Source: three-view drawing plus pictorial views. Frame: mm from the lowest corner of the part. A direction names the side the tool comes from. Give positions to 0.01 mm unless a question says otherwise; leave off trailing zeros. Order: outer loops, then holes, each group sorted by start corner. A loop starts at its lowest first (then second) coordinate and runs counter-clockwise, first axis right, second up. Notation, with made-up numbers: M 38.5,87 L 64.5,87 A23 ccw 64.5,115 Z; hole C 85.5,74 d5. An arc over 180 degrees is marked long. One line per item, written item: value. Start each with the question number.
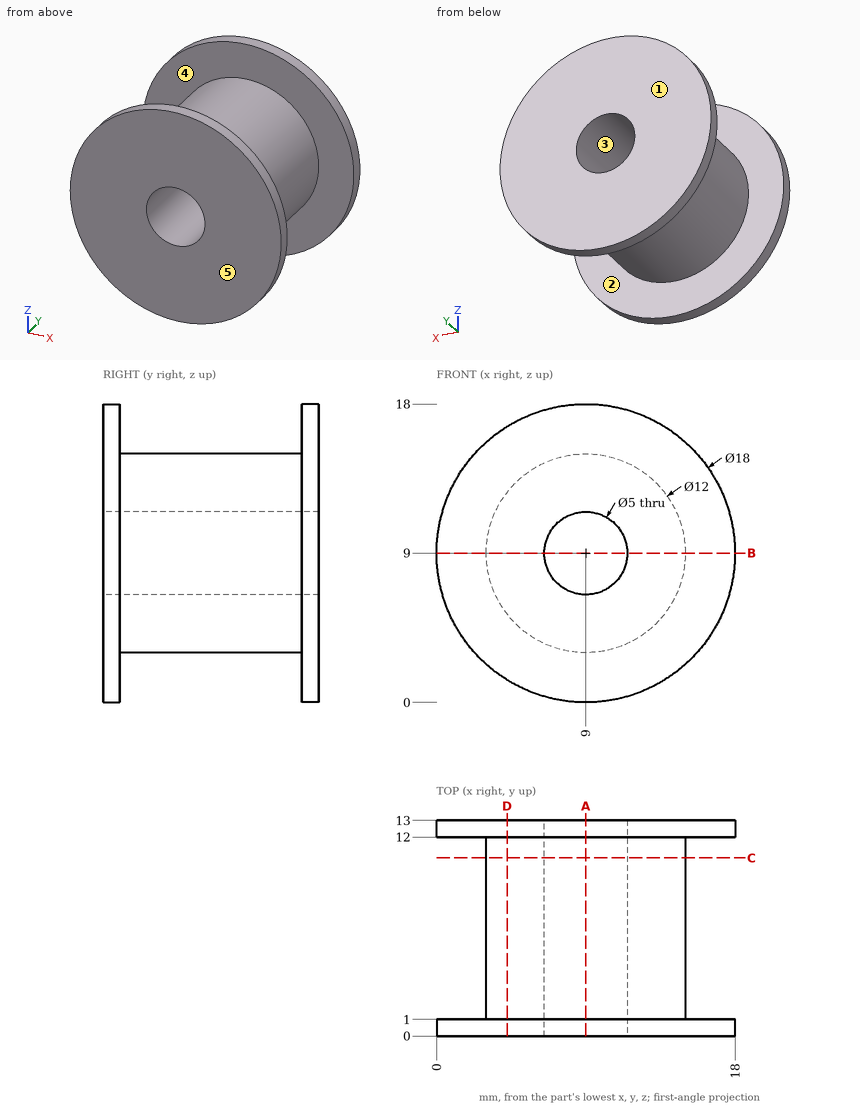
Q1. Set-up query: the marked faces 1 and 2. Return all of +Z, -Z, +X, -X, +Y, -Y with unobstructed straight access to the full face (end or side cutting, diameter ignored); none if empty.
Q2. Section query B-B on z = 9. Return loops of the section in (x, y).
Q3. Mould query, pull axis Y, two halves, no side actions, for the marked faces 3, 4 and 5. Classes: +Y half, -Y half, draft (parallel to the pull), parting line (faces both ways), or undercut.
Q4. Section query D-D on x = 4.25. Return loops of the section in (y, z), and give its area (3 significant figures).
Q5. Contact query for flat-ended pins moving along their axis: pin 1 (5 mm diameter, centred on x = 14.5, y = 10, fed in from -Z); pin 2 (4 mm diameter, centred on x = 4.5, y = 9.5, fed in from +Z); pin 3 (1.5 mm diameter, centred on y = 9.5, z = 4, fed in from +X). Output: stop coordinate, or through.
Q6. Ray query, line 1 along Y through (x, z) = (3.5, 12.75); line 2 along Z through (x, y) = (9, 3.75); line 3 along Z through (x, y) = (10, 2.25). Return the intervals inside material, ascending. Write a range as [from, to].
Q7. Section query C-C on y = 10.75. Return loops of the section in (x, z).
Q8. Section query A-A on x = 9. Return loops of the section in (y, z), and give its area (3 significant figures).
Results below:
1. face 1: +Z, -Z, +X, -X, +Y
1. face 2: none
2. outline: M 0,0 L 6.5,0 L 6.5,13 L 0,13 L 0,12 L 3,12 L 3,1 L 0,1 Z; M 11.5,0 L 18,0 L 18,1 L 15,1 L 15,12 L 18,12 L 18,13 L 11.5,13 Z
3. face 3: draft
3. face 4: undercut
3. face 5: -Y half
4. outline: M 0,1.36 L 1,1.36 L 1,5.33 L 12,5.33 L 12,1.36 L 13,1.36 L 13,16.64 L 12,16.64 L 12,12.67 L 1,12.67 L 1,16.64 L 0,16.64 Z
4. area: 111 mm2
5. pin 1: z = 0.94
5. pin 2: z = 14.45
5. pin 3: x = 13.24
6. line 1: [0, 1], [12, 13]
6. line 2: [3, 6.5], [11.5, 15]
6. line 3: [3.08, 6.71], [11.29, 14.92]
7. outline: C 9,9 d12; hole C 9,9 d5
8. outline: M 0,0 L 1,0 L 1,3 L 12,3 L 12,0 L 13,0 L 13,6.5 L 0,6.5 Z; M 0,11.5 L 13,11.5 L 13,18 L 12,18 L 12,15 L 1,15 L 1,18 L 0,18 Z
8. area: 103 mm2
